```python
from build123d import *

# Parameters (mm, degrees)
F1_DEPTH = 14
F0_R     = 4
F2_DEPTH = 2
F3_R     = 2
F4_SIZE  = 0.6


with BuildPart() as f1:
    # F0 (on Top) → F1 (new body)
    with BuildSketch(Plane.XY):
        with BuildLine():
            ThreePointArc((-31.978437, -6.419222), (-28.055803, -4.219588), (-26.5, 0))
            ThreePointArc((-26.5, 0), (-28.055803, 4.219588), (-31.978437, 6.419222))
            ThreePointArc((-31.978437, 6.419222), (-39.5, 0), (-31.978437, -6.419222))
        make_face()
        with BuildLine():
            ThreePointArc((-31.978437, 6.419222), (-28.055803, 4.219588), (-26.5, 0))
            ThreePointArc((-26.5, 0), (-28.055803, -4.219588), (-31.978437, -6.419222))
            ThreePointArc((-31.978437, -6.419222), (-17.766263, -6.128644), (-4.008308, -9.704817))
            ThreePointArc((-4.008308, -9.704817), (-10.5, 0), (-4.008308, 9.704817))
            ThreePointArc((-4.008308, 9.704817), (-17.766263, 6.128644), (-31.978437, 6.419222))
        make_face()
        with BuildLine():
            ThreePointArc((5.028446, 9.217632), (0.56525, 10.484774), (-4.008308, 9.704817))
            ThreePointArc((-4.008308, 9.704817), (-10.5, 0), (-4.008308, -9.704817))
            ThreePointArc((-4.008308, -9.704817), (0.56525, -10.484774), (5.028446, -9.217632))
            ThreePointArc((5.028446, -9.217632), (9.029083, -5.359632), (10.5, 0))
            ThreePointArc((10.5, 0), (9.029083, 5.359632), (5.028446, 9.217632))
        make_face()
        Polygon((3.752777, 6.5), (7.505553, 0), (3.752777, -6.5), (-3.752777, -6.5), (-7.505553, 0), (-3.752777, 6.5), align=None, mode=Mode.SUBTRACT)
        with BuildLine():
            ThreePointArc((21.007914, 6.423843), (12.788223, 6.505464), (5.028446, 9.217632))
            ThreePointArc((5.028446, 9.217632), (9.029083, 5.359632), (10.5, 0))
            ThreePointArc((10.5, 0), (9.029083, -5.359632), (5.028446, -9.217632))
            ThreePointArc((5.028446, -9.217632), (12.788223, -6.505464), (21.007914, -6.423843))
            ThreePointArc((21.007914, -6.423843), (15.5, 0), (21.007914, 6.423843))
        make_face()
        with BuildLine():
            ThreePointArc((28.5, 0), (26.230924, 4.934499), (21.007914, 6.423843))
            ThreePointArc((21.007914, 6.423843), (15.5, 0), (21.007914, -6.423843))
            ThreePointArc((21.007914, -6.423843), (26.230924, -4.934499), (28.5, 0))
        make_face()
    extrude(amount=F1_DEPTH)

    # F0 (on Top) → F2 (join)
    with BuildSketch(Plane.XY):
        Polygon((3.752777, -6.5), (7.505553, 0), (3.752777, 6.5), (-3.752777, 6.5), (-7.505553, 0), (-3.752777, -6.5), align=None)
        Circle(F0_R, mode=Mode.SUBTRACT)
    extrude(amount=F2_DEPTH)

    # F3
    f3_edges = [f1.edges().sort_by_distance(p)[0] for p in [
        (-17.766263, -6.128644, 14),
    ]]
    fillet(f3_edges, radius=F3_R)

    # F4
    f4_edges = [f1.edges().sort_by_distance(p)[0] for p in [
        (-5.629165, 3.25, 14),
        (0, 6.5, 14),
        (5.629165, 3.25, 14),
        (5.629165, -3.25, 14),
        (0, -6.5, 14),
        (-5.629165, -3.25, 14),
    ]]
    chamfer(f4_edges, length=F4_SIZE)


solid = f1.part
```
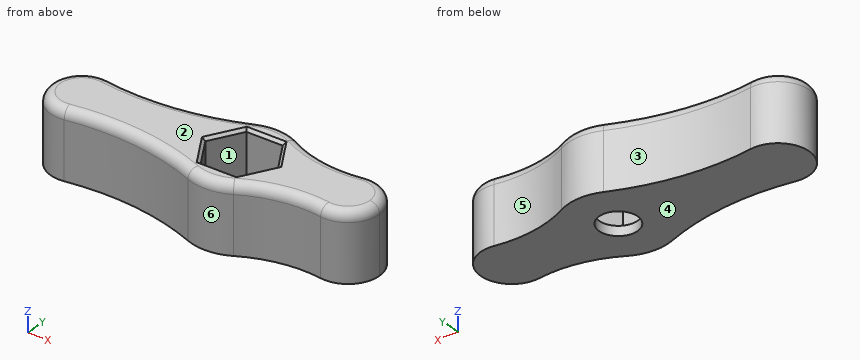
CAD build for the part. Positions are in the model's coordinates, mm. Face numbers are marked on the shaded views. A direction names the side the tool comes from. Give positions to 0.01 mm unless a question says otherwise; leave off trailing zeros. Order: outer loops, then holes, each group sorted by start corner. A loop starts at its lowest first (then second) coordinate and runs counter-clockwise, first axis right, second up. Notation, with made-up numbers: M 51,81 L 91,81 A25 ccw 91,113 Z; hole C 20,52.25 d2. An arc over 180 degrees is marked long. Put each result on its own line as item: value. Start each with the question number.
(1) Saw through at A-A, the plane z = 9.5. Write the cut outline in (x, y).
(2) Mould opens along X. For the marked faces 3, 4, 5 and 6 say: +X half, -X half, draft (parallel to the pull), parting line (faces both ways), or undercut.
(3) Which spindle directions (+Z, -Z, +X, -X, +Y, -Y) get a long thin tool onto all of the face, cutting with end or side? Do the marked faces 1 and 2. Say none if no direction does.
(4) Drill centre lines: line 1 along Y through (x, z) = (0, 1.5); line 2 along X through (y, z) = (-1, 9); line 3 along Z through (x, y) = (6.5, -0.75). Where is each one in solid material? Low to high.
(5) Flat gauge pins, fed straight in: pin 1 Ø6 at (x, z) = (-4, 10) entering from -Y; pin 2 Ø8 at (y, z) = (6.5, 2.5) entering from +X; pin 3 Ø1.5 at (y, z) = (-4.5, 11) entering from +X; pin 4 Ø8 at (y, z) = (-4, 7) entering from -X. Where does each tip first touch, or does it go through?
Check result:
1. outline: M -31.98,-6.42 A51.9 cw -4.01,-9.7 A10.5 ccw 5.03,-9.22 A25.3 cw 21.01,-6.42 A6.5 ccw long 21.01,6.42 A25.3 cw 5.03,9.22 A10.5 ccw -4.01,9.7 A51.9 cw -31.98,6.42 A6.5 ccw long Z; hole M -7.51,0 L -3.75,-6.5 L 3.75,-6.5 L 7.51,0 L 3.75,6.5 L -3.75,6.5 Z
2. face 3: undercut
2. face 4: draft
2. face 5: undercut
2. face 6: parting line
3. face 1: +Z
3. face 2: +Z, +X, -X, +Y, -Y
4. line 1: y = -10.5 to -4, 4 to 10.5
4. line 2: x = -39.42 to -6.93, 6.93 to 28.42
4. line 3: z = 0 to 2
5. pin 1: stops at y = -10.45
5. pin 2: stops at x = 28
5. pin 3: stops at x = 27.31
5. pin 4: stops at x = -39.5
